Check sheet for the drawn part. Datum: minimum x, y, z corner. Units: mm. A direction names the side the tool comes from. Give positions to 0.01 mm unless a question says otherwise; leave off trailing zeros. Loops run counter-clockwise (first coordinate to the right, second up) from the corner with the lowest first, then second, coordinate; pieces in that order, holes last.
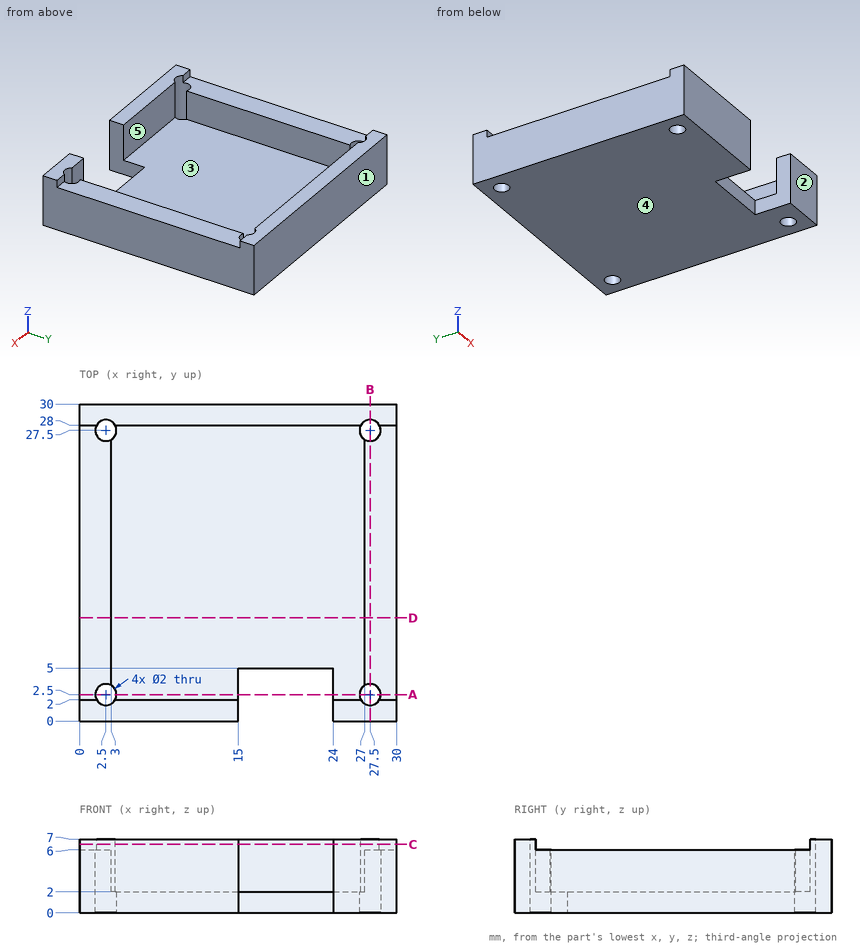
1) Sectioned sample at C-C on z = 6.5. Enter the section's corners in (x, y).
2) Sectioned sample at D-D on y = 9.75. Enter the section's corners in (x, z).
3) Sectioned sample at A-A on y = 2.5. Enter the section's corners in (x, z), plus the area to 3 significant figures.
4) Scan lines: line 1 along Y through (x, z) = (27.5, 4.75); line 2 along X through (y, z) = (2.5, 1.75); line 3 along X through (y, z) = (27, 1). Record each from-to range of solid material in increasing order.
5) Tool access check on the marked faces 4 and 5. Record the directions out of +Z, -Z, +X, -X, +Y, -Y that give a thin tool (end or side, any length) a straight path to the whole face; none if there is none.
6) Mould release check, pull along Y, two halves, no side actions. Record for the marked faces 1, 2 and 3: +Y half, -Y half, draft (parallel to the pull), parting line (faces both ways), or undercut.
7) Depth check by flat-ended pin: P1, Ø0.9, axis at x = 1.5, y = 15.5, coming from the +Z side; P2, Ø0.6, axis at x = 17.5, z = 1, coming from the -Y side; P3, Ø12, axis at x = 17, y = 16, coming from the +Z side. Enter the tip coordinate at first touch or a pass-through.
8) Sectioned sample at B-B on x = 27.5. Enter the section's corners in (y, z).
Determined:
1. outline: (0, 0) - (15, 0) - (15, 2) - (3.37, 2) arc R1 cw to (1.63, 2) - (0, 2) - close; (0, 28) - (1.63, 28) arc R1 cw to (3.37, 28) - (26.63, 28) arc R1 cw to (28.37, 28) - (30, 28) - (30, 30) - (0, 30) - close; (24, 0) - (30, 0) - (30, 2) - (28.37, 2) arc R1 cw to (26.63, 2) - (24, 2) - close
2. outline: (0, 0) - (30, 0) - (30, 6) - (27, 6) - (27, 2) - (3, 2) - (3, 6) - (0, 6) - close
3. outline: (0, 0) - (1.5, 0) - (1.5, 6) - (0, 6) - close; (3.5, 0) - (15, 0) - (15, 2) - (3.5, 2) - close; (24, 0) - (26.5, 0) - (26.5, 2) - (24, 2) - close; (28.5, 0) - (30, 0) - (30, 6) - (28.5, 6) - close
3. area: 46.0 mm2
4. line 1: y = 0 to 1.5, 3.5 to 26.5, 28.5 to 30
4. line 2: x = 0 to 1.5, 3.5 to 15, 24 to 26.5, 28.5 to 30
4. line 3: x = 0 to 1.63, 3.37 to 26.63, 28.37 to 30
5. face 4: -Z, +X, -X, +Y, -Y
5. face 5: +Z
6. face 1: +Y half
6. face 2: -Y half
6. face 3: undercut
7. P1: stops at z = 6
7. P2: stops at y = 5
7. P3: stops at z = 2
8. outline: (0, 0) - (1.5, 0) - (1.5, 7) - (0, 7) - close; (3.5, 0) - (26.5, 0) - (26.5, 6) - (3.5, 6) - close; (28.5, 0) - (30, 0) - (30, 7) - (28.5, 7) - close
